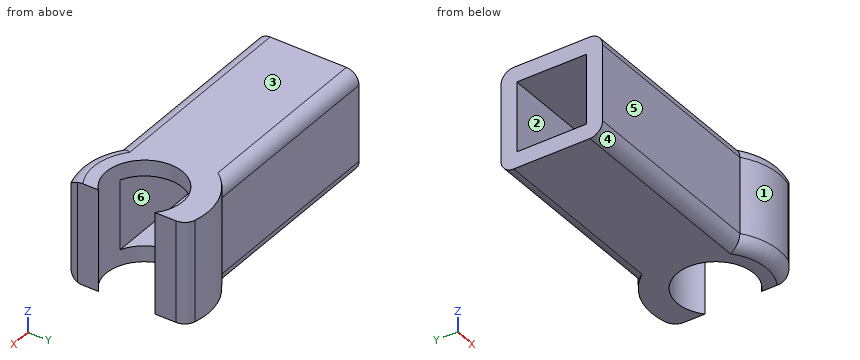
from build123d import *

# Parameters (mm, degrees)
F1_DEPTH = 8
F2_W     = 5.5
F2_H     = 5.5
F3_DEPTH = 17.3020421192
F4_R     = 1


# Not quite as in the source:
# - a feature names something its author has since deleted; it is built from what else it names


with BuildPart() as f1:
    # F0 (on Top) → F1 (new body)
    with BuildSketch(Plane.XY):
        with BuildLine():
            ThreePointArc((2, -2.2360679775), (-3, 0), (2, 2.2360679775))
            Line((2, 2.2360679775), (2, 4.582575695))
            ThreePointArc((2, 4.582575695), (-0.5786610494, 4.9664022582), (-3, 4))
            ThreePointArc((-3, 4), (-5, 0), (-3, -4))
            ThreePointArc((-3, -4), (-0.5786610494, -4.9664022582), (2, -4.582575695))
            Line((2, -4.582575695), (2, -2.2360679775))
        make_face()
        with BuildLine():
            ThreePointArc((-3, -4), (-5, 0), (-3, 4))
            Line((-3, 4), (-18.5, 4))
            Line((-18.5, 4), (-18.5, -4))
            Line((-18.5, -4), (-3, -4))
        make_face()
    extrude(amount=F1_DEPTH)

    # F2 (on face) → F3 (cut, through all)
    with BuildSketch(Plane(origin=(-18.5, 0, 0), x_dir=(0, -1, 0), z_dir=(-1, 0, 0))):
        with Locations((0, 4)):
            Rectangle(F2_W, F2_H)
    extrude(amount=-F3_DEPTH, mode=Mode.SUBTRACT)

    # F4
    f4_edges = [f1.edges().sort_by_distance(p)[0] for p in [
        (2, 4.582576, 4),
        (2, -4.582576, 4),
        (-10.75, -4, 0),
        (-10.75, 4, 8),
        (-10.75, 4, 0),
        (-10.75, -4, 8),
        (-0.578661, -4.966402, 8),
        (-0.578661, -4.966402, 0),
    ]]
    fillet(f4_edges, radius=F4_R)


solid = f1.part
Could you check a few things on this model? Use its own coordinates, in mm. Face numbers are marked on the shaded views. A direction names the side the tool comes from. Coordinates: 2 decimals unless noted, no trailing zeros. Loops run counter-clockwise (first coordinate to the right, second up) from the corner with the lowest first, then second, coordinate; pieces in that order, holes last.
1. Imagine slicing it at D-D (x = -3.5). Please give me the cut outline in (y, z).
2. We'd pull the mould along Y, two halves only. Please class the marked faces 1, 2 and 3: released by +Y, released by -Y, zero draft, split by the parting line, or undercut.
3. For P1, Ø3, axis at x = -12.5, z = 3.5, coming from the +Y side; P2, Ø1.6, axis at x = -10, z = 3, coming from the -Y side; P3, Ø5, axis at x = 0, y = 0, coming from the +Z side, each with a flat end and sliding along its axis, tell me the tip position at first contact or that it passes through.
4. Imagine slicing it at C-C (x = -8.75). Please give me the cut outline in (y, z).
5. For the marked faces 4, 5 and 6, which set-ups out of +Z, -Z, +X, -X, +Y, -Y let a thin tool reach every point of the face, with its end or its side?
6. Imagine slicing it at A-A (z = 3.75). Please give me the cut outline in (x, y), and give its area (3 significant figures).
7. I need wall thicknesses on L1, parallel to Y at x = 0, z = 4; L2, parallel to Y at x = -3, z = 2.75; L3, parallel to Z at x = -7.25, y = -0.75. Which ranges of each line are inside material? Lowest first, please.
8. Imagine slicing it at B-B (y = 0). Please give me the cut outline in (x, z), and give its area (4 significant figures).
Computed values:
1. outline: (-4, 1) arc R1 ccw to (-3, 0) - (3.57, 0) - (3.57, 0.18) arc R1 ccw to (4, 1) - (4, 7) arc R1 ccw to (3.57, 7.82) - (3.57, 8) - (-3, 8) arc R1 ccw to (-4, 7) - close; hole (-2.75, 1.25) - (2.75, 1.25) - (2.75, 6.75) - (-2.75, 6.75) - close
2. face 1: released by -Y
2. face 2: undercut
2. face 3: zero draft
3. P1: stops at y = 4
3. P2: stops at y = -4
3. P3: passes through
4. outline: (-4, 1) arc R1 ccw to (-3, 0) - (3, 0) arc R1 ccw to (4, 1) - (4, 7) arc R1 ccw to (3, 8) - (-3, 8) arc R1 ccw to (-4, 7) - close; hole (-2.75, 1.25) - (2.75, 1.25) - (2.75, 6.75) - (-2.75, 6.75) - close
5. face 4: -Z, -X, -Y
5. face 5: +Z, -Z, -X, -Y
5. face 6: -X
6. outline: (-18.5, -4) - (-3, -4) arc R5 ccw to (1.25, -4.84) arc R1 ccw to (2, -3.87) - (2, -2.24) arc R3 cw to (-1.2, -2.75) - (-18.5, -2.75) - close; (-18.5, 2.75) - (-1.2, 2.75) arc R3 cw to (2, 2.24) - (2, 3.87) arc R1 ccw to (1.25, 4.84) arc R5 ccw to (-3, 4) - (-18.5, 4) - close
6. area: 58.1 mm2
7. L1: y = -5 to -3, 3 to 5
7. L2: y = -4 to -2.75, 2.75 to 4
7. L3: z = 0 to 1.25, 6.75 to 8
8. outline: (-18.5, 0) - (-3, 0) - (-3, 1.25) - (-18.5, 1.25) - close; (-18.5, 6.75) - (-3, 6.75) - (-3, 8) - (-18.5, 8) - close
8. area: 38.75 mm2
